```python
from build123d import *

# Parameters (mm, degrees)
F0_R     = 11.712963
F0_R_2   = 11.53605
F1_DEPTH = 124.714
F2_W     = 87.013735
F2_H     = 97.314427
F3_DEPTH = 28.480272
F4_W     = 86.64881
F4_H     = 97.130336
F5_DEPTH = 28.480272


with BuildPart() as f1:
    # F0 (on Front) → F1 (new body)
    with BuildSketch(Plane.XZ):
        with BuildLine():
            ThreePointArc((-28.479272, -48.582289), (0, -77.061562), (28.479272, -48.582289))
            Line((28.479272, -48.582289), (28.479272, 48.582289))
            ThreePointArc((28.479272, 48.582289), (0, 77.061562), (-28.479272, 48.582289))
            Line((-28.479272, 48.582289), (-28.479272, -48.582289))
        make_face()
        with Locations((0, -48.582289)):
            Circle(F0_R, mode=Mode.SUBTRACT)
        with Locations((0, 48.582289)):
            Circle(F0_R_2, mode=Mode.SUBTRACT)
    extrude(amount=-F1_DEPTH)

    # F2 (on Right) → F3 (cut, through all)
    with BuildSketch(Plane.YZ):
        with Locations((60.919331, 28.530205)):
            Rectangle(F2_W, F2_H)
    extrude(amount=-F3_DEPTH, mode=Mode.SUBTRACT)

    # F4 (on Right) → F5 (cut, through all)
    with BuildSketch(Plane.YZ):
        with Locations((59.381513, 29.164385)):
            Rectangle(F4_W, F4_H)
    extrude(amount=F5_DEPTH, mode=Mode.SUBTRACT)


solid = f1.part
```
Check sheet for the modelled part. Datum: model origin and axes. Units: mm. A direction names the side the tool comes from. Round coordinates to 2 decimals unless told otherwise and drop trailing zeros. Order: outer loops, then holes, each group sorted by start corner. A loop starts at its lowest first (then second) coordinate and runs counter-clockwise, first axis right, second up. Notation, with made-up numbers: M 9,-7 L 18,-7 A36 cw 18,27 Z; hole C 88,69.5 d9. An arc over 180 degrees is marked long. Answer in a Markdown table with one row per item.
(1) Section check A-A on y = 58.5. Record the boundary of the cut face in (x, z).
Findings:
| item | result |
|---|---|
| outline | M -28.48,-48.58 A28.48 ccw 28.48,-48.58 L 28.48,-19.4 L 0,-19.4 L 0,-20.13 L -28.48,-20.13 Z; hole C 0,-48.58 d23.43 |
(2) Set-up check for faces 5 (the cylindrical face through (0.626, 8.584, 77.055)), 6 (the flat face through (14, 102.706, 28)), 7 (the flat face through (-14, 60, -20.127)): record each of +Z, -Z, +X, -X, +Y, -Y from which the full face is reachable in a straight line by a thin tool's end or side.
Findings:
| item | result |
|---|---|
| face 5 | +Z, +Y, -Y |
| face 6 | +Z, +X, -X |
| face 7 | +Z, -X |
(3) Material ranges on line 1 along Z through (x, y) = (0, 3.5); line 2 along Y through (x, z) = (6.5, -18); line 3 along Y through (x, z) = (-12, 49.5), recorded low to high. Write a range as from..to.
Findings:
| item | result |
|---|---|
| line 1 | z = -77.06..-60.3, -36.87..37.05, 60.12..77.06 |
| line 2 | y = 0..16.06, 102.71..124.71 |
| line 3 | y = 0..17.41, 104.43..124.71 |
(4) Gauge pin test, flat ends, axial feed: pin 1 (0.5 mm diameter, centred on y = 104, z = 69, fed in from -X); pin 2 (8.5 mm diameter, centred on x = -15.5, y = 41, fed in from +Z); pin 3 (14 mm diameter, centred on x = 17, y = 76, fed in from +Z). Record the tip position at first contact, or that the pin passes through.
Findings:
| item | result |
|---|---|
| pin 1 | stops at x = 0 |
| pin 2 | stops at z = -20.13 |
| pin 3 | stops at z = -19.4 |
(5) Section check C-C on x = -3. Record the boundary of the cut face in (y, z), plus the area to 3 significant figures.
Findings:
| item | result |
|---|---|
| outline | M 0,-76.9 L 124.71,-76.9 L 124.71,-59.9 L 0,-59.9 Z; M 0,-37.26 L 124.71,-37.26 L 124.71,37.44 L 104.43,37.44 L 104.43,-20.13 L 17.41,-20.13 L 17.41,37.44 L 0,37.44 Z; M 0,59.72 L 17.41,59.72 L 17.41,76.9 L 0,76.9 Z; M 104.43,59.72 L 124.71,59.72 L 124.71,76.9 L 104.43,76.9 Z |
| area | 7,070 mm^2 |
(6) Draft check along Z on faces 1 (the cylindrical face through (10.656, 113.556, 44.164)), 2 (the cylindrical face through (-0.626, 61.484, -77.055)), 3 (the flat face through (14, 16.057, 28)), 4 (the cylindrical face through (-2.539, 61.484, -60.017)). Enter one of: +Z half, -Z half, draft (parallel to the pull), parting line (faces both ways), or undercut.
Findings:
| item | result |
|---|---|
| face 1 | undercut |
| face 2 | -Z half |
| face 3 | draft |
| face 4 | undercut |
(7) Section check B-B on z = -1.5. Record the boundary of the cut face in (x, y), plus the area to 3 significant figures.
Findings:
| item | result |
|---|---|
| outline | M -28.48,0 L 28.48,0 L 28.48,16.06 L 0,16.06 L 0,17.41 L -28.48,17.41 Z; M -28.48,104.43 L 0,104.43 L 0,102.71 L 28.48,102.71 L 28.48,124.71 L -28.48,124.71 Z |
| area | 2,160 mm^2 |
(8) Section check D-D on x = 24. Record the boundary of the cut face in (y, z), plus the area to 3 significant figures.
Findings:
| item | result |
|---|---|
| outline | M 0,-63.91 L 124.71,-63.91 L 124.71,63.91 L 102.71,63.91 L 102.71,-19.4 L 16.06,-19.4 L 16.06,63.91 L 0,63.91 Z |
| area | 8,720 mm^2 |
